```python
from build123d import *

# Parameters (mm, degrees)
SKETCH1_R                   = 25
SKETCH1_R_2                 = 15
SKETCH1_R_3                 = 10
BOSS_EXTRUDE1_DEPTH         = 3
BOSS_EXTRUDE2_DEPTH         = 35
BOSS_EXTRUDE2_DEPTH_BACK    = 110
SKETCH1_3_R                 = 15
SKETCH1_3_R_2               = 10
SKETCH1_4_R                 = 37.5
SKETCH1_4_R_2               = 25
BOSS_EXTRUDE3_DEPTH         = 3
M3_TAPPED_HOLE1_D           = 2.5
M3_TAPPED_HOLE1_CSINK_D     = 3.05
M3_TAPPED_HOLE1_CSINK_ANGLE = 90
SKETCH4_R                   = 15
SKETCH4_R_2                 = 12.5
CUT_EXTRUDE1_DEPTH          = 35
BOSS_EXTRUDE4_DEPTH         = 30


with BuildPart() as part:
    # Sketch1 → Boss-Extrude1 (new body)
    # profile 1 of 2: a face of its own
    with BuildSketch(Plane(origin=(0, 0, 0), x_dir=(0, 0, -1), z_dir=(1, 0, 0))):
        Circle(SKETCH1_R)
        Circle(SKETCH1_R_2, mode=Mode.SUBTRACT)
    # profile 2 of 2: a face of its own
    with BuildSketch(Plane(origin=(0, 0, 0), x_dir=(0, 0, -1), z_dir=(1, 0, 0))):
        Circle(SKETCH1_R_2)
        Circle(SKETCH1_R_3, mode=Mode.SUBTRACT)
    extrude(amount=-BOSS_EXTRUDE1_DEPTH)



with BuildPart() as body_2:
    # Sketch1_3 → Boss-Extrude2 (new, two sides: drawn at the far end of the back side and taken through both)
    with BuildSketch(Plane(origin=(0, 0, 0), x_dir=(0, 0, -1), z_dir=(1, 0, 0)).offset(-BOSS_EXTRUDE2_DEPTH_BACK)):
        Circle(SKETCH1_3_R)
        Circle(SKETCH1_3_R_2, mode=Mode.SUBTRACT)
    extrude(amount=BOSS_EXTRUDE2_DEPTH + BOSS_EXTRUDE2_DEPTH_BACK)


with BuildPart() as part_1:
    add(part.part)

    add(body_2.part)  # Boss-Extrude3 merges body 2
    # Sketch1_4 → Boss-Extrude3 (add)
    with BuildSketch(Plane(origin=(0, 0, 0), x_dir=(0, 0, -1), z_dir=(1, 0, 0))):
        Circle(SKETCH1_4_R)
        Circle(SKETCH1_4_R_2, mode=Mode.SUBTRACT)
    extrude(amount=-BOSS_EXTRUDE3_DEPTH)

    # M3 Tapped Hole1 (through all)
    with Locations(Plane.ZY.offset(3)):
        with Locations((35, 0), (0, 35), (-35, 0), (0, -35), (24.748737342, 24.748737342), (-24.748737342, 24.748737342), (-24.748737342, -24.748737342), (24.748737342, -24.748737342)):
            CounterSinkHole(M3_TAPPED_HOLE1_D / 2, M3_TAPPED_HOLE1_CSINK_D / 2, counter_sink_angle=M3_TAPPED_HOLE1_CSINK_ANGLE)

    # Sketch4 → Cut-Extrude1 (cut)
    with BuildSketch(Plane.ZY.offset(110)):
        with Locations(Location((0, 0, 0), (0, 0, 180))):
            Circle(SKETCH4_R)
        Circle(SKETCH4_R_2, mode=Mode.SUBTRACT)
    extrude(amount=-CUT_EXTRUDE1_DEPTH, mode=Mode.SUBTRACT)

    # Sketch4_3 → Boss-Extrude4 (add)
    with BuildSketch(Plane.ZY.offset(110)):
        with BuildLine():
            Line((4, 15), (-4, 15))
            Line((-4, 15), (-4, 11.842719282))
            ThreePointArc((-4, 11.842719282), (0, 12.5), (4, 11.842719282))
            Line((4, 11.842719282), (4, 15))
        make_face()
        with BuildLine():
            ThreePointArc((12.5, 0), (10.155048006, 7.288689869), (4, 11.842719282))
            Line((4, 11.842719282), (4, -11.842719282))
            ThreePointArc((4, -11.842719282), (10.155048006, -7.288689869), (12.5, 0))
        make_face()
        with BuildLine():
            ThreePointArc((4, 11.842719282), (0, 12.5), (-4, 11.842719282))
            Line((-4, 11.842719282), (-4, -11.842719282))
            ThreePointArc((-4, -11.842719282), (0, -12.5), (4, -11.842719282))
            Line((4, -11.842719282), (4, 11.842719282))
        make_face()
        with BuildLine():
            Line((-4, -11.842719282), (-4, 11.842719282))
            ThreePointArc((-4, 11.842719282), (-12.5, 0), (-4, -11.842719282))
        make_face()
    extrude(amount=-BOSS_EXTRUDE4_DEPTH)


solid = part_1.part
```
The model under review builds one solid part; all positions refer to its coordinate system, in mm. A direction names the side the tool comes from. Round coordinates to 2 decimals unless told otherwise and drop trailing zeros. Order: outer loops, then holes, each group sorted by start corner. A loop starts at its lowest first (then second) coordinate and runs counter-clockwise, first axis right, second up. Notation, with made-up numbers: (-11, 58) -> (-4, 58) arc R17 ccw to (-4, 71) -> close; hole circle Ø6 at (6.5, 46). An arc over 180 degrees is marked (long way). Use a Markdown table: item, result.
Q1. For line 1 (Z direction, x = 1, y = 0); line 2 (X direction, y = -11, z = -19); line 3 (Y direction, x = -51, z = -5.5), list the stretches that pass through material, from the lowest coordinate up.
Values:
| item | result |
|---|---|
| line 1 | z = -15 to -10, 10 to 15 |
| line 2 | x = -3 to 0 |
| line 3 | y = -13.96 to -8.35, 8.35 to 13.96 |
Q2. We need section D-D on y = -18. Write out the cut boundary in (x, z), then the cut area to 3 significant figures.
Values:
| item | result |
|---|---|
| outline | (-3, -32.9) -> (0, -32.9) -> (0, 32.9) -> (-3, 32.9) -> close |
| area | 197 mm^2 |
Q3. Tool access review of faces 4 (the flat face through (0, 1, -16)), 5 (the cylindrical face through (-1.48, 37.18, 4.88)), 6 (the flat face through (-95, 13, -4)): name each direction out of +Z, -Z, +X, -X, +Y, -Y from which nothing blocks a thin tool from reaching the whole face with its end or side.
Values:
| item | result |
|---|---|
| face 4 | +X |
| face 5 | +X, -X |
| face 6 | -Z, -X, +Y |
Q4. Mouldability with a two-part tool opening along Y and no side actions: class faces 1 (the flat face through (-95, 15, 0)), 2 (the flat face through (-95, 13, 4)), 3 (the flat face through (-80, 0, 0)) as +Y half, -Y half, draft (parallel to the pull), parting line (faces both ways), or undercut.
Values:
| item | result |
|---|---|
| face 1 | +Y half |
| face 2 | draft |
| face 3 | undercut |
Q5. Clearance check with flat-ended pins moving along their axes: P1, Ø1.5, axis at y = 15.5, z = 6, coming from the +X side; P2, Ø2, axis at x = -94, z = 1, coming from the -Y side; P3, Ø3, axis at x = 16, z = 6.5, coming from the -Y side. State where each tip first meets the part, or that it passes through.
Values:
| item | result |
|---|---|
| P1 | stops at x = 0 |
| P2 | stops at y = -12.5 |
| P3 | stops at y = -14.14 |
Q6. We need section A-A on x = -55.5. Write out the cut boundary in (y, z), then the cut area to 3 significant figures.
Values:
| item | result |
|---|---|
| outline | circle Ø30 at (0, 0); hole circle Ø20 at (0, 0) |
| area | 393 mm^2 |
Q7. We need section C-C on y = 6. Write out the cut boundary in (x, z).
Values:
| item | result |
|---|---|
| outline | (-110, -10.97) -> (-75, -10.97) -> (-75, -13.75) -> (-3, -13.75) -> (-3, -37.02) -> (0, -37.02) -> (0, -13.75) -> (35, -13.75) -> (35, -8) -> (-80, -8) -> (-80, 8) -> (35, 8) -> (35, 13.75) -> (0, 13.75) -> (0, 37.02) -> (-3, 37.02) -> (-3, 13.75) -> (-75, 13.75) -> (-75, 10.97) -> (-110, 10.97) -> close |
Q8. We need section B-B on y = -8.5. Write out the cut boundary in (x, z).
Values:
| item | result |
|---|---|
| outline | (-110, -9.17) -> (-75, -9.17) -> (-75, -12.36) -> (-3, -12.36) -> (-3, -36.52) -> (0, -36.52) -> (0, -12.36) -> (35, -12.36) -> (35, -5.27) -> (-80, -5.27) -> (-80, 5.27) -> (35, 5.27) -> (35, 12.36) -> (0, 12.36) -> (0, 36.52) -> (-3, 36.52) -> (-3, 12.36) -> (-75, 12.36) -> (-75, 9.17) -> (-110, 9.17) -> close |
